from build123d import *

# Parameters (mm, degrees)
F1_DEPTH    = 10.16
F2_T2_ANGLE = 284.1697303729


# Not quite as in the source:
# - a fillet or chamfer that OpenCascade refuses, or shapes differently, is made with other operations: its cross-section is extruded or revolved along the edge and cut away or added


with BuildPart() as f1:
    # F0 (on Front) → F1 (new body)
    with BuildSketch(Plane.XZ):
        with BuildLine():
            Line((-116.84, 0), (0, 0))
            Line((0, 0), (0, 57.15))
            Line((0, 57.15), (-2.6989761401, 57.15))
            ThreePointArc((-2.6989761401, 57.15), (-58.42, 12.7), (-114.1410238599, 57.15))
            Line((-114.1410238599, 57.15), (-116.84, 57.15))
            Line((-116.84, 57.15), (-116.84, 0))
        make_face()
    extrude(amount=F1_DEPTH)

    # F2: chamfer of 24.892 x 4.3891312038 on 1 edges, made by hand

    # F2_s1 → F2_t2 (revolve, cut)
    with BuildSketch(Plane(origin=(-70.2228677722, 0, 54.6968082658), x_dir=(0, 1, 0), z_dir=(-0.7889217924, 0, 0.6144936171))):
        Polygon((14.732, -76.3574700932), (-10.16, -80.746601297), (-10.16, -76.3574700932), align=None)
    revolve(axis=Axis((-58.42, -10.16, 69.85), (0, 1, 0)), revolution_arc=F2_T2_ANGLE, mode=Mode.SUBTRACT)


solid = f1.part
Geometry check sheet. Reference: the model listing, model coordinates, mm. Coordinates: 2 decimals unless noted, no trailing zeros. Order: outer loops, then holes, each group sorted by start corner. A loop starts at its lowest first (then second) coordinate and runs counter-clockwise, first axis right, second up. Notation, with made-up numbers: (1.5, 36.5) - (47.5, 36.5) arc R20 cw to (47.5, 55.5) - close; hole circle Ø3 at (57, 55). An arc over 180 degrees is marked (long way). Answer in a Markdown table with one row per item. Add a question column.
1) Gauge pin test, flat end, axial feed: P1, Ø6, axis at x = -90.5, y = -1.5, coming from the +Z side. Record the tip position at first contact, or that the pin passes through.
2) Cross-section at A-A, the plane y = -4. Record the cut outline in (x, z), then the cut area to 3 significant figures.
3) Material ranges on line 1 along X through (y, z) = (-1.25, 18); line 2 along X through (y, z) = (-7, 18); line 3 along Z through (x, y) = (-80, -6), recorded low to high. Write a range as [from, to].
Check result:
| question | item | result |
|---|---|---|
| 1 | P1 | stops at z = 21.25 |
| 2 | outline | (-116.84, 0) - (0, 0) - (0, 54.3) arc R60.45 cw to (-116.84, 54.3) - close |
| 2 | area | 2,460 mm² |
| 3 | line 1 | x = [-116.84, -88.55], [-28.29, 0] |
| 3 | line 2 | x = [-116.84, -90.52], [-26.32, 0] |
| 3 | line 3 | z = [0, 13] |
